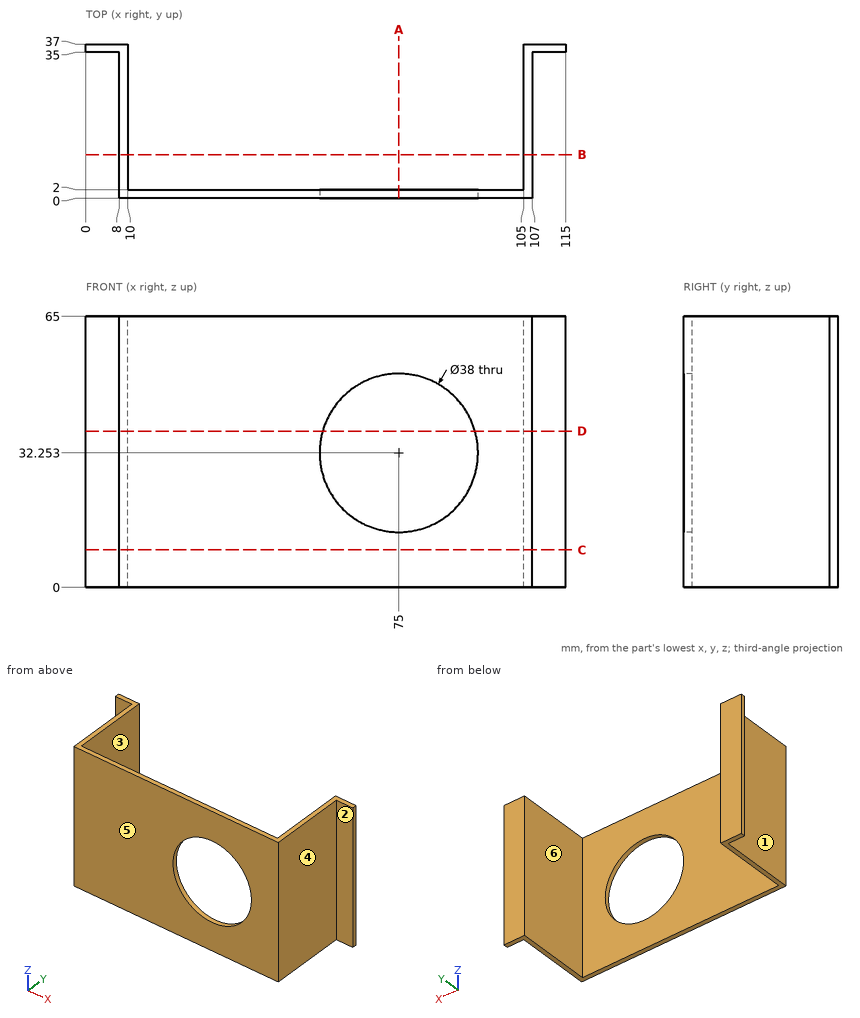
Print and shaded views of the part. All mm, measured from the part's lowest x, y and z. A direction names the side the tool comes from. Round coordinates to 2 decimals unless told otherwise and drop trailing zeros. Write each loop counter-clockwise with the first axis right and the second up, starting at its lowest first coordinate (ties: lowest second). Pieces come first, ordered by that corner, then holes. Notation, with made-up numbers: (-17, 32) -> (28, 32) arc R9 ccw to (28, 49) -> close; hole circle Ø2 at (13, 11). An arc over 180 degrees is marked (long way). Write item = value, one per line.
(1) Band-saw the part on D-D (z = 37.5). Give the cut face in (x, y), then the cut area to 3 significant figures.
Answer:
outline = (0, 35) -> (8, 35) -> (8, 0) -> (56.74, 0) -> (56.74, 2) -> (10, 2) -> (10, 37) -> (0, 37) -> close; (93.26, 0) -> (107, 0) -> (107, 35) -> (115, 35) -> (115, 37) -> (105, 37) -> (105, 2) -> (93.26, 2) -> close
area = 297 mm2
(2) Tool access for the marked faces 4, 5 and 6: list every direction of +Z, -Z, +X, -X, +Y, -Y with a clear straight run to the whole face (end or side of a thin tool).
Answer:
face_4 = +Z, -Z, +X, -Y
face_5 = +Z, -Z, +X, -X, -Y
face_6 = +Z, -Z, +Y
(3) Flat gauge pins, fed straight in: pin 1 (10 mm diameter, centred on y = 7.5, z = 19.5, fed in from +X); pin 2 (2 mm diameter, centred on y = 31.5, z = 19, fed in from -X); pin 3 (4 mm diameter, centred on x = 109.5, z = 17.5, fed in from -Y). Where does each tip first touch, or does it go through?
Answer:
pin_1 = 107
pin_2 = 8
pin_3 = 35
(4) Two-plate mould, pull along X, no slides. Class the marked faces 1, 2 and 3: pulls with the +X half, pulls with the -X half, needs draft (parallel to the pull), parting line crosses it, or undercut.
Answer:
face_1 = pulls with the -X half
face_2 = needs draft
face_3 = undercut
(5) Probe L1, parallel to Z at x = 75, y = 1; L2, parallel to X at y = 14.5, z = 49; L3, parallel to Y at x = 35.5, z = 28.5. List the from-to ranges inside material, lowest first.
Answer:
L1 = 0 to 13.25, 51.25 to 65
L2 = 8 to 10, 105 to 107
L3 = 0 to 2
(6) Band-saw the part on B-B (y = 10.5). Give the cut face in (x, z), then the cut area to 3 significant figures.
Answer:
outline = (8, 0) -> (10, 0) -> (10, 65) -> (8, 65) -> close; (105, 0) -> (107, 0) -> (107, 65) -> (105, 65) -> close
area = 260 mm2
(7) Band-saw the part on C-C (z = 9). Give the cut face in (x, y), then the cut area to 3 significant figures.
Answer:
outline = (0, 35) -> (8, 35) -> (8, 0) -> (107, 0) -> (107, 35) -> (115, 35) -> (115, 37) -> (105, 37) -> (105, 2) -> (10, 2) -> (10, 37) -> (0, 37) -> close
area = 370 mm2
(8) Band-saw the part on A-A (x = 75). Give the cut face in (y, z).
Answer:
outline = (0, 0) -> (2, 0) -> (2, 13.25) -> (0, 13.25) -> close; (0, 51.25) -> (2, 51.25) -> (2, 65) -> (0, 65) -> close
